```python
from build123d import *

# Parameters (mm, degrees)
SKETCH4_W               = 63.5
SKETCH4_H               = 50.8
BOSS_EXTRUDE2_DEPTH     = 5.08
F_1_4_CLEARANCE_HOLE2_D = 6.7564
BOSS_EXTRUDE3_DEPTH     = 20.828
M3_CLEARANCE_HOLE1_D    = 3.4
CUT_EXTRUDE1_DEPTH      = 20.828
FILLET2_R               = 4.318
SKETCH13_W              = 68.58
SKETCH13_H              = 55.88
SKETCH13_W_2            = 63.5
SKETCH13_H_2            = 50.8
BOSS_EXTRUDE4_DEPTH     = 5.08
FILLET3_R               = 7.62
FILLET4_R               = 1.27


with BuildPart() as part:
    # Sketch4 → Boss-Extrude2 (new body)
    with BuildSketch(Plane(origin=(0, 0, 0), x_dir=(1, 0, 0), z_dir=(0, 1, 0))):
        Rectangle(SKETCH4_W, SKETCH4_H)
    extrude(amount=BOSS_EXTRUDE2_DEPTH)

    # 1/4 Clearance Hole2 (through all)
    with Locations(Plane(origin=(-25.4, 5.08, -19.05), x_dir=(0, 0, 1), z_dir=(0, 1, 0))):
        with Locations((0, 0), (0, 50.8), (38.1, 50.8), (38.1, 0)):
            Hole(F_1_4_CLEARANCE_HOLE2_D / 2)

    # Sketch7 → Boss-Extrude3 (add)
    with BuildSketch(Plane(origin=(0, 5.08, 0), x_dir=(1, 0, 0), z_dir=(0, 1, 0))):
        Polygon((0, 22.86), (22.86, 0), (0, -22.86), (-22.86, 0), align=None)
    extrude(amount=BOSS_EXTRUDE3_DEPTH)

    # M3 Clearance Hole1 (through all)
    with Locations(Plane(origin=(0, 25.908, -9.525), x_dir=(0, 0, 1), z_dir=(0, 1, 0))):
        with Locations((0, 0), (9.525, 9.525), (19.05, 0), (9.525, -9.525)):
            Hole(M3_CLEARANCE_HOLE1_D / 2)

    # Sketch12 → Cut-Extrude1 (cut)
    with BuildSketch(Plane(origin=(0, 0, 0), x_dir=(-1, 0, 0), z_dir=(0, -1, 0))):
        Polygon((0, -19.05), (-19.05, 0), (0, 19.05), (19.05, 0), align=None)
    extrude(amount=-CUT_EXTRUDE1_DEPTH, mode=Mode.SUBTRACT)

    # Fillet2
    fillet2_edges = [part.edges().sort_by_distance(p)[0] for p in [
        (-11.43, 5.08, -11.43),
        (0, 15.494, -22.86),
        (-11.43, 5.08, 11.43),
        (-22.86, 15.494, 0),
        (11.43, 5.08, 11.43),
        (0, 15.494, 22.86),
        (11.43, 5.08, -11.43),
        (22.86, 15.494, 0),
        (-11.43, 25.908, -11.43),
        (-11.43, 25.908, 11.43),
        (11.43, 25.908, 11.43),
        (11.43, 25.908, -11.43),
    ]]
    fillet(fillet2_edges, radius=FILLET2_R)

    # Sketch13 → Boss-Extrude4 (add)
    with BuildSketch(Plane.XZ):
        Rectangle(SKETCH13_W, SKETCH13_H)
        Rectangle(SKETCH13_W_2, SKETCH13_H_2, mode=Mode.SUBTRACT)
    extrude(amount=-BOSS_EXTRUDE4_DEPTH)

    # Fillet3
    fillet3_edges = [part.edges().sort_by_distance(p)[0] for p in [
        (-34.29, 2.54, -27.94),
        (-34.29, 2.54, 27.94),
        (34.29, 2.54, 27.94),
        (34.29, 2.54, -27.94),
    ]]
    fillet(fillet3_edges, radius=FILLET3_R)

    # Fillet4
    fillet4_edges = [part.edges().sort_by_distance(p)[0] for p in [
        (0, 5.08, 27.94),
        (-34.29, 5.08, 0),
        (34.29, 5.08, 0),
        (0, 5.08, -27.94),
        (32.058153673, 5.08, -25.708153673),
        (32.058153673, 5.08, 25.708153673),
        (-32.058153673, 5.08, -25.708153673),
        (-32.058153673, 5.08, 25.708153673),
    ]]
    fillet(fillet4_edges, radius=FILLET4_R)


solid = part.part
```
Here's how the part is built. I have some questions about the finished solid (model axes, mm). A direction names the side the tool comes from. Give positions to 0.01 mm unless a question says otherwise; leave off trailing zeros. Order: outer loops, then holes, each group sorted by start corner. A loop starts at its lowest first (then second) coordinate and runs counter-clockwise, first axis right, second up. Notation, with made-up numbers: (29.5, -6.75) - (48.5, -6.75) arc R31 cw to (48.5, 31.25) - close; hole circle Ø9 at (-4, 23.25). An arc over 180 degrees is marked (long way). Answer as a JSON object with one key per item and string values. Group by question number.
Item 1: If we section it at A-A on y = 12.5: Please give me the cut outline in (x, z).
Item 2: If we section it at B-B on y = 7.5: Please give me the cut outline in (x, z).
Item 3: For P1, Ø8, axis at y = 21, z = -12, coming from the +X side; P2, Ø8, axis at x = 25.4, z = -19.05, coming from the +Y side; P3, Ø3, axis at y = 13, z = 5.5, coming from the +X side, each with a flat end and sliding along its axis, tell me the tip position at first contact or that it passes through.
Item 4: If we mould it in two halves opening along Z, with no side actions, what happens to faces 1 (the cylindrical face through (22.4, 2.5, -20.6)), 2 (the cylindrical face through (-28.7, 2.5, -18.32)), 3 (the cylindrical face through (31.999, 1.932, -25.767)), 4 (the cylindrical face through (-12.47, 6.31, 12.23))? For each: pulls with the +Z half, pulls with the -Z half, needs draft (parallel to the pull), parting line crosses it, or undercut.
Item 5: Please list where these lines run through material, in increasing order: probe 1 along X at (y, z) = (22.25, 0) (3 decimals); probe 2 along X at (y, z) = (24.55, 0) (3 decimals); probe 3 along X at (y, z) = (19, -2).
Item 6: Which directions (+Z, -Z, +X, -X, +Y, -Y) give clear straight access to the entire face, cutting with the end or side of a thin tool? Please do faces 5 (the cylindrical face through (-21.07, 15.58, -0.05)), 6 (the flat face through (11.31, 15.41, -11.55)), 7 (the flat face through (-11.31, 15.41, 11.55)).
Result set:
{
 "1": {"outline": "(-19.81, -3.05) - (-3.05, -19.81) arc R4.32 ccw to (3.05, -19.81) - (19.81, -3.05) arc R4.32 ccw to (19.81, 3.05) - (3.05, 19.81) arc R4.32 ccw to (-3.05, 19.81) - (-19.81, 3.05) arc R4.32 ccw to start; hole (-19.05, 0) - (0, -19.05) - (19.05, 0) - (0, 19.05) - close"},
 "2": {"outline": "(-20.12, -3.36) - (-3.36, -20.12) arc R4.76 ccw to (3.36, -20.12) - (20.12, -3.36) arc R4.76 ccw to (20.12, 3.36) - (3.36, 20.12) arc R4.76 ccw to (-3.36, 20.12) - (-20.12, 3.36) arc R4.76 ccw to start; hole (-19.05, 0) - (0, -19.05) - (19.05, 0) - (0, 19.05) - close"},
 "3": {"P1": "x = 14.86", "P2": "y = 5.08", "P3": "x = 18.86"},
 "4": {"face 1": "undercut", "face 2": "undercut", "face 3": "pulls with the -Z half", "face 4": "pulls with the +Z half"},
 "5": {"probe 1": "-21.021 to -11.225, -7.825 to 7.825, 11.225 to 21.021", "probe 2": "-19.897 to -11.225, -7.825 to 7.825, 11.225 to 19.897", "probe 3": "-20.58 to -17.05, 17.05 to 20.58"},
 "6": {"face 5": "-X, +Y", "face 6": "-Z, +X, +Y", "face 7": "+Z, -X, +Y"}
}
